```python
from build123d import *

# Parameters (mm, degrees)
SKETCH1_R           = 3
BOSS_EXTRUDE1_DEPTH = 25
SKETCH2_R           = 5
BOSS_EXTRUDE2_DEPTH = 1
CHAMFER1_SIZE       = 0.6
CHAMFER2_SIZE       = 0.2


with BuildPart() as part:
    # Sketch1 → Boss-Extrude1 (new body)
    with BuildSketch(Plane.XY):
        Circle(SKETCH1_R)
    extrude(amount=BOSS_EXTRUDE1_DEPTH)

    # Sketch2 → Boss-Extrude2 (add)
    with BuildSketch(Plane.XY.offset(25)):
        Circle(SKETCH2_R)
    extrude(amount=BOSS_EXTRUDE2_DEPTH)

    # Chamfer1
    chamfer1_edges = [part.edges().sort_by_distance(p)[0] for p in [
        (-3, 0, 0),
    ]]
    chamfer(chamfer1_edges, length=CHAMFER1_SIZE)

    # Chamfer2
    chamfer2_edges = [part.edges().sort_by_distance(p)[0] for p in [
        (-5, 0, 26),
    ]]
    chamfer(chamfer2_edges, length=CHAMFER2_SIZE)


solid = part.part
```
Geometry check sheet. Reference: the model listing, model coordinates, mm. A direction names the side the tool comes from. Coordinates: 2 decimals unless noted, no trailing zeros. Order: outer loops, then holes, each group sorted by start corner. A loop starts at its lowest first (then second) coordinate and runs counter-clockwise, first axis right, second up.
Item 1: Tool access check on faces 1 (the flat face through (-0.1, -3.3, 25)), 2 (the flat face through (0, 0, 0)). Record the directions out of +Z, -Z, +X, -X, +Y, -Y that give a thin tool (end or side, any length) a straight path to the whole face; none if there is none.
Item 2: Depth check by flat-ended pin: pin 1 (2 mm diameter, centred on x = 4, y = -0.5, fed in from -Z); pin 2 (1 mm diameter, centred on x = 2, z = 19.5, fed in from -Y); pin 3 (5 mm diameter, centred on y = 0, z = 12.5, fed in from -X). Enter the tip coordinate at first touch or a pass-through.
Item 3: Scan lines: line 1 along Z through (x, y) = (3.25, -2.75); line 2 along X through (y, z) = (1, 10); line 3 along X through (y, z) = (2.25, 13.25). Record each from-to range of solid material in increasing order.
Item 4: Section check A-A (y = 0). Enter the section's corners in (x, z).
Item 5: Section check C-C (z = 19.25). Enter the section's corners in (x, y), plus the area to 3 significant figures.
Check sheet entries:
1. face 1: -Z
1. face 2: -Z, +X, -X, +Y, -Y
2. pin 1: stops at z = 25
2. pin 2: stops at y = -2.6
2. pin 3: stops at x = -3
3. line 1: z = 25 to 26
3. line 2: x = -2.83 to 2.83
3. line 3: x = -1.98 to 1.98
4. outline: (-5, 25) - (-3, 25) - (-3, 0.6) - (-2.4, 0) - (2.4, 0) - (3, 0.6) - (3, 25) - (5, 25) - (5, 25.8) - (4.8, 26) - (-4.8, 26) - (-5, 25.8) - close
5. outline: circle Ø6 at (0, 0)
5. area: 28.3 mm2
